Autodesk Inventor part; units mm, degrees
ref_plane "YZ Plane" through (0, 0, 0) normal (1, 0, 0) x (0, 1, 0)
ref_plane "XZ Plane" through (0, 0, 0) normal (0, 1, 0) x (-1, 0, 0)
ref_plane "XY Plane" through (0, 0, 0) normal (0, 0, 1) x (1, 0, 0)
sketch "Sketch1" plane through (0, 0, 0) normal (0, 1, 0) x (-1, 0, 0)
  circle A0 centre (0, 0) radius 22.5
  dimension "d0" = 45
extrude "Extrusion1" add sketch "Sketch1" along normal blind 25
sketch "Sketch2" plane through (0, 25, 0) normal (0, 1, 0) x (1, 0, 0)
  circle A0 centre (0, 0) radius 19.0081
extrude "Extrusion2" add sketch "Sketch2" along normal blind 9
sketch "Sketch3" plane through (0, 34, 0) normal (0, 1, 0) x (1, 0, 0)
  circle A0 centre (0, 0) radius 22.5
extrude "Extrusion3" add sketch "Sketch3" along normal blind 30
sketch "Sketch4" plane through (0, 64, 0) normal (0, 1, 0) x (1, 0, 0)
  circle A0 centre (0, 0) radius 5
  dimension "d7" = 10
extrude "Extrusion4" add sketch "Sketch4" along normal blind 25
sketch "Sketch5" plane through (0, 0, 0) normal (0, -1, 0) x (1, 0, 0)
  circle A0 centre (0, 11.2132) radius 5.0141
  circle A1 centre (0, -12.5914) radius 5.0157
  point P0 (0, 0)
extrude "Extrusion5" add sketch "Sketch5" along normal blind 25
properties part number "DC motor now"
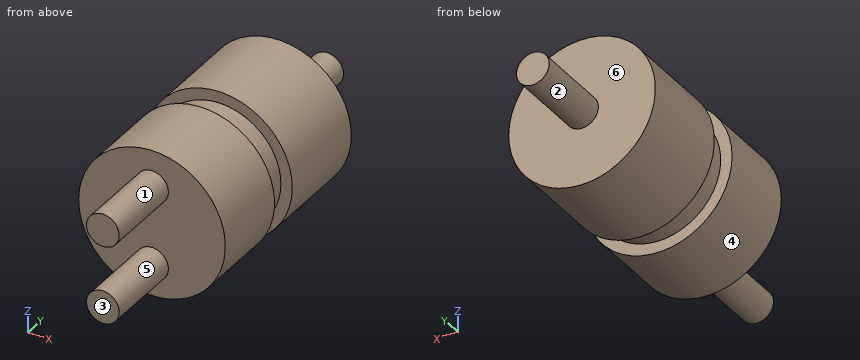
Source: CAD feature listing. Evaluate the final solid. Frame: model axes, mm. Face numbers are marked on the shaded views. A direction names the side the tool comes from. Round coordinates to 2 decimals unless told otherwise and drop trailing zeros. Loops run counter-clockwise (first coordinate to the right, second up) from the corner with the lowest first, then second, coordinate; pieces in that order, holes last. Notation, with made-up numbers: M 19.5,-6.75 L 50.5,-6.75 A15 cw 50.5,-2.75 Z; hole C 76.5,67 d6. An arc over 180 degrees is marked long. Return JSON: item names as keys, results as strings. Group by question number.
1. Section query D-D on x = -10. Output: boundary loops of the cut face in (y, z), and give its area (3 significant figures).
2. Section query A-A on x = 0. Output: boundary loops of the cut face in (y, z), and give its area (3 significant figures).
3. Pin query (flat end, axial travel): pin 1 (12 mm diameter, centred on y = 6, z = 12, fed in from +X); pin 2 (1.5 mm diameter, centred on x = 8, z = 12.5, fed in from -Y); pin 3 (2 mm diameter, centred on x = 1, y = 17.5, fed in from +Z); pin 4 (13.5 mm diameter, centred on x = 7, z = -7.5, fed in from -Y). Return the tip coordinate at first contact, or that it passes through.
4. Material intervals for line 1 along Y through (x, z) = (-4.5, -8); line 2 along Y through (x, z) = (10.5, 16.5); line 3 along X through (y, z) = (44, 1), sorted ascending. Write a range as from..to.
5. Section query B-B on z = 0. Output: boundary loops of the cut face in (x, y), and give its area (3 significant figures).
6. Section query C-C on y = 22.5. Output: boundary loops of the cut face in (x, z), and give its area (3 significant figures).
7. Reachability of the marked faces 1, 2 and 3 from +Z, -Z, +X, -X, +Y, -Y: full face, straight path, thin tool, end or side. Return the list, or none.
8. Mould query, pull axis Z, two halves, no side actions, for the marked faces 4, 5 and 6. Classes: released by +Z, released by -Z, zero draft, split by the parting line, or undercut.
Checks:
{
 "1": {"outline": "M 0,-20.16 L 25,-20.16 L 25,-16.17 L 34,-16.17 L 34,-20.16 L 64,-20.16 L 64,20.16 L 34,20.16 L 34,16.17 L 25,16.17 L 25,20.16 L 0,20.16 Z", "area": "2,510 mm²"},
 "2": {"outline": "M -25,-17.61 L 0,-17.61 L 0,-22.5 L 25,-22.5 L 25,-19.01 L 34,-19.01 L 34,-22.5 L 64,-22.5 L 64,-5 L 89,-5 L 89,5 L 64,5 L 64,22.5 L 34,22.5 L 34,19.01 L 25,19.01 L 25,22.5 L 0,22.5 L 0,16.23 L -25,16.23 L -25,6.2 L 0,6.2 L 0,-7.58 L -25,-7.58 Z", "area": "3,570 mm²"},
 "3": {"pin 1": "stops at x = 21.69", "pin 2": "stops at y = 0", "pin 3": "stops at z = 22.5", "pin 4": "stops at y = -25"},
 "4": {"line 1": "y = 0..64", "line 2": "y = 0..25, 34..64", "line 3": "x = -22.48..22.48"},
 "5": {"outline": "M -22.5,0 L 22.5,0 L 22.5,25 L 19.01,25 L 19.01,34 L 22.5,34 L 22.5,64 L 5,64 L 5,89 L -5,89 L -5,64 L -22.5,64 L -22.5,34 L -19.01,34 L -19.01,25 L -22.5,25 Z", "area": "3,070 mm²"},
 "6": {"outline": "C 0,0 d45", "area": "1,590 mm²"},
 "7": {"face 1": "-Y", "face 2": "+Y", "face 3": "+Z, -Z, +X, -X, -Y"},
 "8": {"face 4": "split by the parting line", "face 5": "undercut", "face 6": "zero draft"}
}
